Read the model definition and answer for the solid it produces. Units are mm, in the model's axes. A direction names the side the tool comes from. Coordinates: 2 decimals unless noted, no trailing zeros. Order: outer loops, then holes, each group sorted by start corner. A loop starts at its lowest first (then second) coordinate and runs counter-clockwise, first axis right, second up.
from build123d import *

# Parameters (mm, degrees)
SKETCH_1_R      = 1.5
EXTRUDE_4_DEPTH = 1


with BuildPart() as part:
    # 草图1 → 凸台-拉伸4 (new body)
    with BuildSketch(Plane(origin=(0, 0, 0), x_dir=(1, 0, 0), z_dir=(0, 1, 0))):
        Polygon((-17.435269168, 2.881354455), (16.393730682, 2.881354455), (20.235837144, 0), (-0.520769243, -22.484942941), (-21.903688145, 0), align=None)
        with Locations((-17.435269168, 0)):
            Circle(SKETCH_1_R, mode=Mode.SUBTRACT)
        with Locations((16.393730682, 0)):
            Circle(SKETCH_1_R, mode=Mode.SUBTRACT)
        Polygon((-14.435269168, 0), (0, 0), (13.393730682, 0), (-0.520769243, -14.366164827), align=None, mode=Mode.SUBTRACT)
    extrude(amount=EXTRUDE_4_DEPTH)


solid = part.part
Q1. Which of the six approach directions +Z, -Z, +X, -X, +Y, -Y give full straight-line access (tool end or side, diameter ignored) to faces 1 (the flat face through (-0.7, 0.5, 0)), 2 (the flat face through (18.29, 0.49, -1.46))?
Q2. The part is cut by section A-A, the plane x = -18.5. Determine the outline of the cut face in (y, z), then the cut area to 3 significant figures.
Q3. Straight lines are drawn through the part: L1, parallel to X at y = 0.2, z = -1.25; L2, parallel to Z at x = 8, y = 0.2; L3, parallel to X at y = 0.75, z = 6.5. For each, find the intervals that lie inside material, in ascending order.
Q4. Determine the mould class of faces 3 (the flat face through (10, 0.49, 11.09)), 4 (the flat face through (-7.381, 0.493, 7.284)), 5 (the flat face through (-19.7, 0.49, -1.42)), 6 (the flat face through (-0.8, 0.5, -2.881)) for opening direction X: +X half, -X half, draft (parallel to the pull), parting line (faces both ways), or undercut.
Q5. This flat-tipped pin is pushed along its axis until it touches: P1, Ø12, axis at x = -4.5, z = 6, coming from the +Y side. Where does it stop, or does it pass through?
Q6. The part is cut by section C-C, the plane y = 0.85. Determine the outline of the cut face in (x, z), then the cut area to 3 significant figures.
Q7. The part is cut by section B-B, the plane z = 13.5. Determine the outline of the cut face in (x, y).
Q8. The part is cut by section D-D, the plane z = 0.5. Determine the outline of the cut face in (x, y), then the cut area to 3 significant figures.
Computed values:
1. face 1: +Y, -Y
1. face 2: -Z, +X, +Y, -Y
2. outline: (0, -2.19) - (1, -2.19) - (1, -1.06) - (0, -1.06) - close; (0, 1.06) - (1, 1.06) - (1, 3.58) - (0, 3.58) - close
2. area: 3.66 mm2
3. L1: x = -19.97 to -18.26, -16.61 to 15.56, 17.22 to 18.57
3. L2: z = -2.88 to 0, 5.57 to 13.25
3. L3: x = -15.72 to -8.14, 7.1 to 14.24
4. face 3: +X half
4. face 4: undercut
4. face 5: -X half
4. face 6: draft
5. P1: stops at y = 1
6. outline: (-21.9, 0) - (-17.44, -2.88) - (16.39, -2.88) - (20.24, 0) - (-0.52, 22.48) - close; hole circle Ø3 at (-17.44, 0); hole (-14.44, 0) - (13.39, 0) - (-0.52, 14.37) - close; hole circle Ø3 at (16.39, 0)
6. area: 369 mm2
7. outline: (-9.07, 0) - (-1.36, 0) - (-1.36, 1) - (-9.07, 1) - close; (0.32, 0) - (7.77, 0) - (7.77, 1) - (0.32, 1) - close
8. outline: (-21.43, 0) - (-18.85, 0) - (-18.85, 1) - (-21.43, 1) - close; (-16.02, 0) - (-13.95, 0) - (-13.95, 1) - (-16.02, 1) - close; (12.91, 0) - (14.98, 0) - (14.98, 1) - (12.91, 1) - close; (17.81, 0) - (19.77, 0) - (19.77, 1) - (17.81, 1) - close
8. area: 8.69 mm2
